Geometry: see drawing. Coordinates: mm, zero at the bounding-box minimum. Coordinates: 2 decimals unless noted, no trailing zeros. Write each loop counter-clockwise with the first axis right and the second up, starting at its lowest first coordinate (ties: lowest second). Pieces come first, ordered by that corner, then holes.
1) Section query A-A (z = 1.45). State how many separate pieces and enclosed holes the cut face has, then the cut area to 3 significant figures.
2) Line query: L1, parallel to X at y = 2.75, z = 1.65; L2, parallel to X at y = 6.5, z = 2.8; L3, parallel to X at y = 3.25, z = 2. Output: solid intervals per line, ascending.
3) Section query B-B (x = 143). Output: boundary loops of the cut face in (y, z).
4) Pin query (flat end, axial travel): pin 1 Ø0.7 at (y, z) = (9, 1.5) entering from +X; pin 2 Ø0.9 at (x, z) = (213, 1) entering from -Y; pin 3 Ø0.9 at (x, z) = (49.5, 2) entering from -Y. Return the tip coordinate at first contact, or that it passes through.
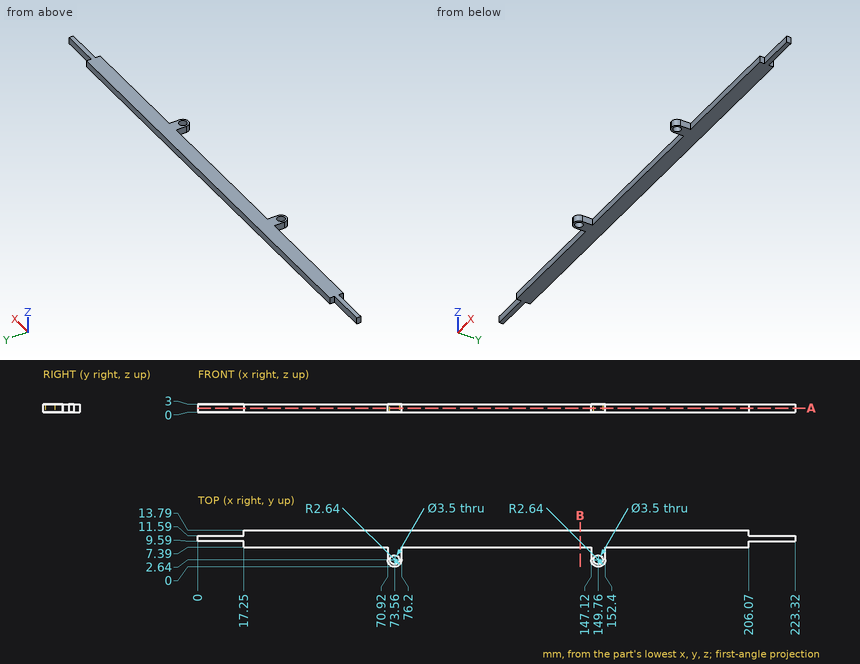
Answer:
1. separate pieces: 1
1. enclosed holes: 2
1. area: 1,330 mm2
2. L1: x = 70.92 to 71.81, 75.31 to 76.2, 147.12 to 148.01, 151.51 to 152.4
2. L2: x = 70.92 to 76.2, 147.12 to 152.4
2. L3: x = 70.92 to 71.92, 75.2 to 76.2, 147.12 to 148.12, 151.4 to 152.4
3. outline: (7.39, 0) - (13.79, 0) - (13.79, 3) - (7.39, 3) - close
4. pin 1: stops at x = 206.07
4. pin 2: stops at y = 9.59
4. pin 3: stops at y = 7.39
